```python
from build123d import *

# Parameters (mm, degrees)
BODY_DEPTH              = 15
CHAMFER1_SIZE           = 1
F_3_2_3_2_FORSENSOR_D   = 3.2
F_3_2_3_2_FORCARRIAGE_D = 3.2


with BuildPart() as part:
    # Sketch1 → Body (new body)
    with BuildSketch(Plane.XY):
        Polygon((0, 0), (0, 20), (2, 20), (2, 2), (15, 2), (15, 0), align=None)
    extrude(amount=BODY_DEPTH)

    # Chamfer1
    chamfer1_edges = [part.edges().sort_by_distance(p)[0] for p in [
        (1, 20, 15),
        (1, 20, 0),
        (15, 1, 15),
        (15, 1, 0),
    ]]
    chamfer(chamfer1_edges, length=CHAMFER1_SIZE)

    # Ø3.2 (3.2) ForSensor (through all)
    with Locations(Plane(origin=(0, 2, 0), x_dir=(1, 0, 0), z_dir=(0, 1, 0))):
        with Locations((11, -2.775), (11, -12.225)):
            Hole(F_3_2_3_2_FORSENSOR_D / 2)

    # Ø3.2 (3.2) ForCarriage (through all)
    with Locations(Plane(origin=(2, 0, 0), x_dir=(0, 0, -1), z_dir=(1, 0, 0))):
        with Locations((-11.25, 13), (-3.75, 13)):
            Hole(F_3_2_3_2_FORCARRIAGE_D / 2)


solid = part.part
```
Could you check a few things on this model? Use its own coordinates, in mm. A direction names the side the tool comes from. Coordinates: 2 decimals unless noted, no trailing zeros. Order: outer loops, then holes, each group sorted by start corner. A loop starts at its lowest first (then second) coordinate and runs counter-clockwise, first axis right, second up. Notation, with made-up numbers: M 41.25,-32 L 97.25,-32 A25 cw 97.25,6 Z; hole C 24.5,71 d8. An arc over 180 degrees is marked long. Use a Markdown table: item, result. Add a question column.
Q1. I want a section at B-B on y = 13. List the corners of the cut face in (x, z) for me.
Q2. I'm going to push flat-ended pins straight in: pin 1 (7.5 mm diameter, centred on y = 10, z = 8.5, fed in from +X); pin 2 (3 mm diameter, centred on x = 11, z = 2.775, fed in from +Y); pin 3 (4 mm diameter, centred on x = 5.5, z = 9, fed in from +Y). Where does each tip first touch, or does it pass through?
Q3. I want a section at C-C on z = 4.75. List the corners of the cut face in (x, y) for me, then the cut area to 3 significant figures.
Q4. We'd pull the mould along Z, two halves only. Please class faces 1 (the flat face through (1, 19.5, 0.5)), 2 (the flat face through (1, 19.5, 14.5)), 3 (the cylindrical face through (12.6, 1, 12.2)): pulls with the +Z half, pulls with the -Z half, needs draft (parallel to the pull), parting line crosses it, or undercut.
Q5. I want a section at A-A on x = 11. List the corners of the cut face in (y, z) for me (3 decimals), then the cut area to 3 significant figures.
Q6. If I drill on L1, parallel to Z at x = 11, y = 1.1 (3 decimals); L2, parallel to Y at x = 1.45, z = 11.25; L3, parallel to X at y = 18.5, z = 6.25, over which ranges is the centre line in solid material (lowest first)?
Q7. Which directions (+Z, -Z, +X, -X, +Y, -Y) give clear straight access to the entire face, cutting with the end or side of a thin tool? Please do faces 4 (the flat face through (2, 11, 7)), 5 (the flat face through (14.5, 1, 14.5)).
Q8. I want a section at D-D on y = 2.25. List the corners of the cut face in (x, z) for me, then the cut area to 3 significant figures.
Checked values:
| question | item | result |
|---|---|---|
| 1 | outline | M 0,0 L 2,0 L 2,2.15 L 0,2.15 Z; M 0,5.35 L 2,5.35 L 2,9.65 L 0,9.65 Z; M 0,12.85 L 2,12.85 L 2,15 L 0,15 Z |
| 2 | pin 1 | x = 2 |
| 2 | pin 2 | through |
| 2 | pin 3 | y = 2 |
| 3 | outline | M 0,0 L 15,0 L 15,2 L 2,2 L 2,11.75 L 0,11.75 Z; M 0,14.25 L 2,14.25 L 2,20 L 0,20 Z |
| 3 | area | 61.0 mm² |
| 4 | face 1 | pulls with the -Z half |
| 4 | face 2 | pulls with the +Z half |
| 4 | face 3 | undercut |
| 5 | outline | M 0,0 L 2,0 L 2,1.175 L 0,1.175 Z; M 0,4.375 L 2,4.375 L 2,10.625 L 0,10.625 Z; M 0,13.825 L 2,13.825 L 2,15 L 0,15 Z |
| 5 | area | 17.2 mm² |
| 6 | L1 | 0 to 1.175, 4.375 to 10.625, 13.825 to 15 |
| 6 | L2 | 0 to 11.4, 14.6 to 20 |
| 6 | L3 | 0 to 2 |
| 7 | face 4 | +Z, -Z, +X, +Y |
| 7 | face 5 | +Z, +X, +Y, -Y |
| 8 | outline | M 0,0 L 2,0 L 2,15 L 0,15 Z |
| 8 | area | 30.0 mm² |
